CAD build for the part. Positions are in the model's coordinates, mm. Face numbers are marked on the shaded views. A direction names the side the tool comes from. Coordinates: 2 decimals unless noted, no trailing zeros. Order: outer loops, then holes, each group sorted by start corner. A loop starts at its lowest first (then second) coordinate and runs counter-clockwise, first axis right, second up. Notation, with made-up numbers: M -37.75,89.5 L -1.75,89.5 A12 cw -1.75,111.5 Z; hole C -34.5,36.25 d1. An arc over 180 degrees is marked long. Write item = value, one per line.
from build123d import *

# Parameters (mm, degrees)
SALIENTE_EXTRUIR3_DEPTH = 50
CROQUIS37_3_R           = 11
CROQUIS37_3_R_2         = 1.7
SALIENTE_EXTRUIR4_DEPTH = 2.5
CROQUIS38_R             = 17.69
CROQUIS38_R_2           = 16.19
SALIENTE_EXTRUIR5_DEPTH = 4
SALIENTE_EXTRUIR6_START = -1.5
CROQUIS40_R             = 19.19
CROQUIS40_R_2           = 17.69
SALIENTE_EXTRUIR6_DEPTH = 1.5
CROQUIS41_W             = 18.5
CROQUIS41_H             = 10.5
CORTAR_EXTRUIR1_DEPTH   = 11.5
SALIENTE_EXTRUIR7_DEPTH = 3
CROQUIS44_R             = 2.5
CORTAR_EXTRUIR2_DEPTH   = 3


with BuildPart() as part:
    # Croquis37 → Saliente-Extruir3 (new body)
    with BuildSketch(Plane.XY):
        with BuildLine():
            Line((-24.106917755, -16.878527403), (-24.106917755, 16.707259035))
            ThreePointArc((-24.106917755, 16.707259035), (-23.829078048, 18.104053563), (-23.037857506, 19.288198786))
            Line((-23.037857506, 19.288198786), (-19.330750725, 22.995305567))
            ThreePointArc((-19.330750725, 22.995305567), (-18.146605502, 23.78652611), (-16.749810974, 24.064365816))
            Line((-16.749810974, 24.064365816), (16.835975464, 24.064365816))
            ThreePointArc((16.835975464, 24.064365816), (18.232769992, 23.78652611), (19.416915215, 22.995305567))
            Line((19.416915215, 22.995305567), (23.124021997, 19.288198786))
            ThreePointArc((23.124021997, 19.288198786), (23.915242539, 18.104053563), (24.193082245, 16.707259035))
            Line((24.193082245, 16.707259035), (24.193082245, -16.878527403))
            ThreePointArc((24.193082245, -16.878527403), (23.915242539, -18.275321931), (23.124021997, -19.459467154))
            Line((23.124021997, -19.459467154), (19.416915215, -23.166573935))
            ThreePointArc((19.416915215, -23.166573935), (18.232769992, -23.957794478), (16.835975464, -24.235634184))
            Line((16.835975464, -24.235634184), (-16.749810974, -24.235634184))
            ThreePointArc((-16.749810974, -24.235634184), (-18.146605502, -23.957794478), (-19.330750725, -23.166573935))
            Line((-19.330750725, -23.166573935), (-23.037857506, -19.459467154))
            ThreePointArc((-23.037857506, -19.459467154), (-23.829078048, -18.275321931), (-24.106917755, -16.878527403))
        make_face()
        with BuildLine():
            ThreePointArc((16.835975464, -21.235634184), (17.084719695, -21.18615588), (17.295594872, -21.045253592))
            Line((17.295594872, -21.045253592), (21.002701653, -17.338146811))
            ThreePointArc((21.002701653, -17.338146811), (21.143603941, -17.127271634), (21.193082245, -16.878527403))
            Line((21.193082245, -16.878527403), (21.193082245, 16.707259035))
            ThreePointArc((21.193082245, 16.707259035), (21.143603941, 16.956003266), (21.002701653, 17.166878443))
            Line((21.002701653, 17.166878443), (17.295594872, 20.873985224))
            ThreePointArc((17.295594872, 20.873985224), (17.084719695, 21.014887512), (16.835975464, 21.064365816))
            Line((16.835975464, 21.064365816), (-16.749810974, 21.064365816))
            ThreePointArc((-16.749810974, 21.064365816), (-16.998555205, 21.014887512), (-17.209430381, 20.873985224))
            Line((-17.209430381, 20.873985224), (-20.916537162, 17.166878443))
            ThreePointArc((-20.916537162, 17.166878443), (-21.057439451, 16.956003266), (-21.106917755, 16.707259035))
            Line((-21.106917755, 16.707259035), (-21.106917755, -16.878527403))
            ThreePointArc((-21.106917755, -16.878527403), (-21.057439451, -17.127271634), (-20.916537162, -17.338146811))
            Line((-20.916537162, -17.338146811), (-17.209430381, -21.045253592))
            ThreePointArc((-17.209430381, -21.045253592), (-16.998555205, -21.18615588), (-16.749810974, -21.235634184))
            Line((-16.749810974, -21.235634184), (16.835975464, -21.235634184))
        make_face(mode=Mode.SUBTRACT)
    extrude(amount=-SALIENTE_EXTRUIR3_DEPTH)



with BuildPart() as body_2:
    # Croquis37_3 → Saliente-Extruir4 (new body)
    with BuildSketch(Plane.XY):
        with BuildLine():
            Line((16.835975464, -21.235634184), (-16.749810974, -21.235634184))
            ThreePointArc((-16.749810974, -21.235634184), (-16.998555205, -21.18615588), (-17.209430381, -21.045253592))
            Line((-17.209430381, -21.045253592), (-20.916537162, -17.338146811))
            ThreePointArc((-20.916537162, -17.338146811), (-21.057439451, -17.127271634), (-21.106917755, -16.878527403))
            Line((-21.106917755, -16.878527403), (-21.106917755, 16.707259035))
            ThreePointArc((-21.106917755, 16.707259035), (-21.057439451, 16.956003266), (-20.916537162, 17.166878443))
            Line((-20.916537162, 17.166878443), (-17.209430381, 20.873985224))
            ThreePointArc((-17.209430381, 20.873985224), (-16.998555205, 21.014887512), (-16.749810974, 21.064365816))
            Line((-16.749810974, 21.064365816), (16.835975464, 21.064365816))
            ThreePointArc((16.835975464, 21.064365816), (17.084719695, 21.014887512), (17.295594872, 20.873985224))
            Line((17.295594872, 20.873985224), (21.002701653, 17.166878443))
            ThreePointArc((21.002701653, 17.166878443), (21.143603941, 16.956003266), (21.193082245, 16.707259035))
            Line((21.193082245, 16.707259035), (21.193082245, -16.878527403))
            ThreePointArc((21.193082245, -16.878527403), (21.143603941, -17.127271634), (21.002701653, -17.338146811))
            Line((21.002701653, -17.338146811), (17.295594872, -21.045253592))
            ThreePointArc((17.295594872, -21.045253592), (17.084719695, -21.18615588), (16.835975464, -21.235634184))
        make_face()
        with Locations((0.043082245, -0.085634184)):
            Circle(CROQUIS37_3_R, mode=Mode.SUBTRACT)
        with Locations((15.543082245, 15.414365816)):
            Circle(CROQUIS37_3_R_2, mode=Mode.SUBTRACT)
        with Locations((-15.456917755, 15.414365816)):
            Circle(CROQUIS37_3_R_2, mode=Mode.SUBTRACT)
        with Locations((15.543082245, -15.585634184)):
            Circle(CROQUIS37_3_R_2, mode=Mode.SUBTRACT)
        with Locations((-15.456917755, -15.585634184)):
            Circle(CROQUIS37_3_R_2, mode=Mode.SUBTRACT)
    extrude(amount=-SALIENTE_EXTRUIR4_DEPTH)


with BuildPart() as part_1:
    add(part.part)

    add(body_2.part)  # Saliente-Extruir5 merges body 2
    # Croquis38 → Saliente-Extruir5 (add)
    with BuildSketch(Plane.XY):
        with Locations((0.043082245, -0.085634184)):
            Circle(CROQUIS38_R)
        with Locations((0.043082245, -0.085634184)):
            Circle(CROQUIS38_R_2, mode=Mode.SUBTRACT)
    extrude(amount=SALIENTE_EXTRUIR5_DEPTH)

    # Croquis40 → Saliente-Extruir6 (add)
    with BuildSketch(Plane.XY.offset(4).offset(SALIENTE_EXTRUIR6_START)):
        Circle(CROQUIS40_R)
        with Locations((0.043082245, -0.085634184)):
            Circle(CROQUIS40_R_2, mode=Mode.SUBTRACT)
    extrude(amount=SALIENTE_EXTRUIR6_DEPTH)

    # Croquis41 → Cortar-Extruir1 (cut)
    with BuildSketch(Plane.XZ.offset(24.235634184)):
        with Locations((0.045189026, -44.75)):
            Rectangle(CROQUIS41_W, CROQUIS41_H)
    extrude(amount=-CORTAR_EXTRUIR1_DEPTH, mode=Mode.SUBTRACT)

    # Croquis42 → Saliente-Extruir7 (add)
    with BuildSketch(Plane.XZ.offset(24.235634184)):
        with BuildLine():
            Line((-16.749810974, -10), (-28.749810974, -10))
            ThreePointArc((-28.749810974, -10), (-32.749810974, -14), (-28.749810974, -18))
            Line((-28.749810974, -18), (-16.749810974, -18))
            Line((-16.749810974, -18), (-16.749810974, -10))
        make_face()
        with BuildLine():
            Line((16.767018988, -9.971120394), (16.780805296, -17.971108515))
            Line((16.780805296, -17.971108515), (28.780787478, -17.950429053))
            ThreePointArc((28.780787478, -17.950429053), (32.773888384, -13.943541838), (28.767001169, -9.950440932))
            Line((28.767001169, -9.950440932), (16.767018988, -9.971120394))
        make_face()
        with BuildLine():
            Line((-16.749810974, -40), (-28.749810974, -40))
            ThreePointArc((-28.749810974, -40), (-32.749810974, -36), (-28.749810974, -32))
            Line((-28.749810974, -32), (-16.749810974, -32))
            Line((-16.749810974, -32), (-16.749810974, -40))
        make_face()
        with BuildLine():
            Line((16.767018988, -40.028879606), (16.780805296, -32.028891485))
            Line((16.780805296, -32.028891485), (28.780787478, -32.049570947))
            ThreePointArc((28.780787478, -32.049570947), (32.773888384, -36.056458162), (28.767001169, -40.049559068))
            Line((28.767001169, -40.049559068), (16.767018988, -40.028879606))
        make_face()
    extrude(amount=-SALIENTE_EXTRUIR7_DEPTH)

    # Croquis44 → Cortar-Extruir2 (cut)
    with BuildSketch(Plane(origin=(0, -21.235634184, 0), x_dir=(1, 0, 0), z_dir=(0, 1, 0))):
        with Locations(Location((-28.749810974, 36, 0), (0, 0, 180))):
            Circle(CROQUIS44_R)
        with Locations(Location((28.773894323, 36.049565008, 0), (0, 0, 180))):
            Circle(CROQUIS44_R)
        with Locations(Location((28.773894323, 13.950434992, 0), (0, 0, 180))):
            Circle(CROQUIS44_R)
        with Locations(Location((-28.749810974, 14, 0), (0, 0, 180))):
            Circle(CROQUIS44_R)
    extrude(amount=-CORTAR_EXTRUIR2_DEPTH, mode=Mode.SUBTRACT)


solid = part_1.part
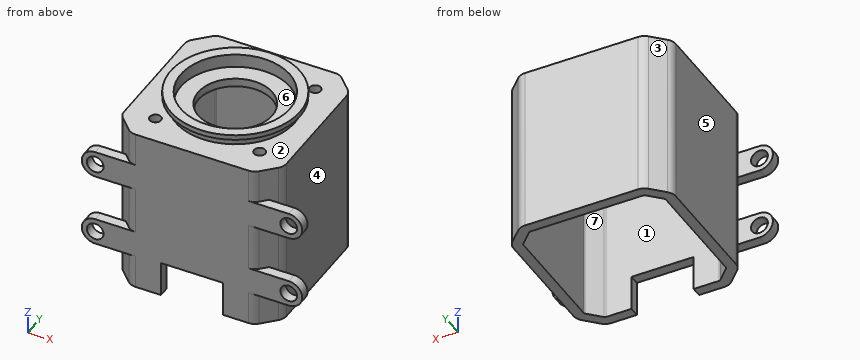
(1) Slice it at D-D, the plane z = -35. State how many separate pieces and enclosed holes the cut face has, then the cut area to 3 significant figures.
Evaluation:
separate_pieces = 3
enclosed_holes = 1
area = 557 mm²
(2) Pin check, flat tips, straight feed: pin 1 Ø4 at (x, z) = (28, -37) entering from +Y; pin 2 Ø1.5 at (x, y) = (1, -23) entering from -Z; pin 3 Ø2 at (x, z) = (-23.5, -27) entering from -Y. Stop position of each tip, or through.
Evaluation:
pin_1 = -21.24
pin_2 = -39.5
pin_3 = -20
(3) Pull direction Y, two halves, no side cores. Call the marked faces 1, 2 and 3: +Y half, -Y half, draft (parallel to the pull), parting line (faces both ways), or undercut.
Evaluation:
face_1 = undercut
face_2 = draft
face_3 = +Y half
(4) Slice it at C-C, the plane y = -12. Write the cut outline in (x, z).
Evaluation:
outline = M -24.11,-50 L -21.11,-50 L -21.11,-2.5 L 21.19,-2.5 L 21.19,-50 L 24.19,-50 L 24.19,0 L 13.12,0 L 13.12,2.5 L 14.98,2.5 L 14.98,4 L 11.01,4 L 11.01,0 L -10.92,0 L -10.92,4 L -14.98,4 L -14.98,2.5 L -13.03,2.5 L -13.03,0 L -24.11,0 Z
(5) Slice it at B-B, the plane x = 0. Write the cut outline in (y, z).
Evaluation:
outline = M -24.24,-39.5 L -21.24,-39.5 L -21.24,-2.5 L -11.09,-2.5 L -11.09,0 L -16.28,0 L -16.28,4 L -19.19,4 L -19.19,2.5 L -17.78,2.5 L -17.78,0 L -24.24,0 Z; M 10.91,-2.5 L 21.06,-2.5 L 21.06,-50 L 24.06,-50 L 24.06,0 L 17.6,0 L 17.6,2.5 L 19.19,2.5 L 19.19,4 L 16.1,4 L 16.1,0 L 10.91,0 Z
(6) Tool access for the marked faces 4, 5, 6 and 7: list every direction of +Z, -Z, +X, -X, +Y, -Y with a clear straight run to the whole face (end or side of a thin tool).
Evaluation:
face_4 = +Z, -Z, +X, +Y
face_5 = +Z, -Z, -X, +Y
face_6 = +Z
face_7 = -Z
(7) Wall check: line 1 (X direction, y = 13, z = -14.5); line 2 (Y direction, x = 1, z = -16); line 3 (X direction, y = -17, z = -1.5). Give the ranges that are in metal, low to high. Write a range as from..to.
Evaluation:
line_1 = -24.11..-21.11, 21.19..24.19
line_2 = -24.24..-21.24, 21.06..24.06
line_3 = -24.1..-16.4, -14.51..14.6, 16.49..24.19
